from build123d import *

# Parameters (mm, degrees)
F1_DEPTH = 19.05
F2_R     = 6.35
F3_R     = 6.35


with BuildPart() as f1:
    # F0 (on Front) → F1 (new body)
    with BuildSketch(Plane.XZ):
        Polygon((0, 76.2), (0, 0), (76.2, 0), (76.2, 12.7), (12.7, 76.2), align=None)
    extrude(amount=F1_DEPTH)

    # F2
    f2_edges = [f1.edges().sort_by_distance(p)[0] for p in [
        (12.7, -9.525, 76.2),
        (76.2, -9.525, 12.7),
    ]]
    fillet(f2_edges, radius=F2_R)

    # F3
    f3_edges = [f1.edges().sort_by_distance(p)[0] for p in [
        (44.45, -19.05, 44.45),
        (44.45, 0, 44.45),
    ]]
    fillet(f3_edges, radius=F3_R)


solid = f1.part
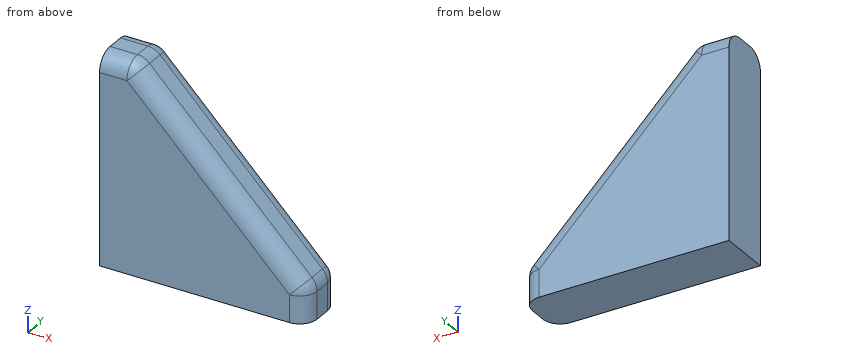
Source: CAD feature listing. Evaluate the final solid. Frame: model axes, mm. Round coordinates to 2 decimals unless told otherwise and drop trailing zeros. Write each loop counter-clockwise with the first axis right and the second up, starting at its lowest first coordinate (ties: lowest second). Pieces come first, ordered by that corner, then holes. Notation, with made-up numbers: (82.5, 59) - (92.5, 59) arc R21 cw to (92.5, 73) - close; hole circle Ø6 at (80, -22). An arc over 180 degrees is marked (long way). Use CSV: the item, a comma, the result in double quotes. Start each with the question number.
(1) Material intervals for probe 1 along X at (y, z) = (-10.75, 10.5); probe 2 along Z at (x, y) = (12.5, -5.75); probe 3 along Z at (x, y) = (52, -11.25), sorted ascending. Write a range as [from, to].
(2) Cut plane B-B, the plane y = -2.25. Return loops of the section in (x, z).
(3) First-contact query: pin 1 Ø6 at (x, y) = (15, -9) entering from +Z; pin 2 Ø10 at (y, z) = (-15, 64) entering from +X; pin 3 Ø8 at (x, y) = (62, -4.5) entering from +Z. Flat tips, straight axial feed; report the tip coordinate or a pass-through.
(4) Cut plane A-A, the plane y = -8.25. Return loops of the section in (x, z), and give its area (3 significant figures).
Geometry says:
1,probe 1,"[0, 76.19]"
1,probe 2,"[0, 75.69]"
1,probe 3,"[0, 36.9]"
2,outline,"(0, 0) - (74.7, 0) - (74.7, 10.07) arc R4.85 ccw to (73.28, 13.5) - (13.5, 73.28) arc R4.85 ccw to (10.07, 74.7) - (0, 74.7) - close"
3,pin 1,"z = 75.9"
3,pin 2,"x = 29.62"
3,pin 3,"z = 30.7"
4,outline,"(0, 0) - (76.2, 0) - (76.2, 10.07) arc R6.35 ccw to (74.34, 14.56) - (14.56, 74.34) arc R6.35 ccw to (10.07, 76.2) - (0, 76.2) - close"
4,area,"3,790 mm²"
